from build123d import *

# Parameters (mm, degrees)
SKETCH_1_R          = 11
SKETCH_1_R_2        = 4.15
EXTRUDE_1_DEPTH     = 2
EXTRUDE_START       = 5
SKETCH_1_3_R        = 5.65
SKETCH_1_3_R_2      = 4.15
EXTRUDE_2_DEPTH     = 5
CUT_EXTRUDE_1_DEPTH = 4
SKETCH_4_R          = 11
SKETCH_4_R_2        = 6.15
EXTRUDE_3_DEPTH     = 10
CUT_EXTRUDE_START   = -8
SKETCH_5_W          = 5.562300803
SKETCH_5_H          = 5
CUT_EXTRUDE_2_DEPTH = 8


with BuildPart() as part:
    # Sketch 1 → Extrude 1 (new body)
    with BuildSketch(Plane(origin=(0, 0, 0), x_dir=(1, 0, 0), z_dir=(0, 1, 0))):
        with Locations(Location((0, 0, 0), (0, 0, 270))):
            Circle(SKETCH_1_R)
        with Locations(Location((0, 0, 0), (0, 0, 270))):
            Circle(SKETCH_1_R_2, mode=Mode.SUBTRACT)
    extrude(amount=-EXTRUDE_1_DEPTH)

    # Sketch 1_3 → Extrude 2 (add)
    with BuildSketch(Plane(origin=(0, 0, 0), x_dir=(1, 0, 0), z_dir=(0, 1, 0)).offset(EXTRUDE_START)):
        with Locations(Location((0, 0, 0), (0, 0, 270))):
            Circle(SKETCH_1_3_R)
        with Locations(Location((0, 0, 0), (0, 0, 270))):
            Circle(SKETCH_1_3_R_2, mode=Mode.SUBTRACT)
    extrude(amount=-EXTRUDE_2_DEPTH)

    # Sketch 2 → Cut-Extrude 1 (cut)
    with BuildSketch(Plane(origin=(0, 5, 0), x_dir=(1, 0, 0), z_dir=(0, 1, 0))):
        with BuildLine():
            Line((1.95, 5.302829433), (1.95, 3.663331817))
            ThreePointArc((1.95, 3.663331817), (4.15, 0), (1.95, -3.663331817))
            Line((1.95, -3.663331817), (1.95, -5.302829433))
            ThreePointArc((1.95, -5.302829433), (5.65, 0), (1.95, 5.302829433))
        make_face()
        with BuildLine():
            Line((-1.95, 5.302829433), (-1.95, 3.663331817))
            ThreePointArc((-1.95, 3.663331817), (-4.15, 0), (-1.95, -3.663331817))
            Line((-1.95, -3.663331817), (-1.95, -5.302829433))
            ThreePointArc((-1.95, -5.302829433), (-5.65, 0), (-1.95, 5.302829433))
        make_face()
    extrude(amount=-CUT_EXTRUDE_1_DEPTH, mode=Mode.SUBTRACT)

    # Sketch 4 → Extrude 3 (add)
    with BuildSketch(Plane.XZ.offset(2)):
        with Locations(Location((0, 0, 0), (0, 0, 90))):
            Circle(SKETCH_4_R)
        with Locations(Location((0, 0, 0), (0, 0, 270))):
            Circle(SKETCH_4_R_2, mode=Mode.SUBTRACT)
    extrude(amount=EXTRUDE_3_DEPTH)

    # Sketch 5 → Cut-Extrude 2 (cut)
    with BuildSketch(Plane.XZ.offset(12).offset(CUT_EXTRUDE_START)):
        with BuildLine():
            ThreePointArc((3.25, 10.508924778), (0, 11), (-3.25, 10.508924778))
            Line((-3.25, 10.508924778), (-3.25, 5.221110993))
            ThreePointArc((-3.25, 5.221110993), (0, 6.15), (3.25, 5.221110993))
            Line((3.25, 5.221110993), (3.25, 10.508924778))
        make_face()
        with Locations((-8.400091582, 0)):
            Rectangle(SKETCH_5_W, SKETCH_5_H)
    extrude(amount=CUT_EXTRUDE_2_DEPTH, mode=Mode.SUBTRACT)


solid = part.part
Geometry check sheet. Reference: the model listing, model coordinates, mm. A direction names the side the tool comes from. Round coordinates to 2 decimals unless told otherwise and drop trailing zeros. Order: outer loops, then holes, each group sorted by start corner. A loop starts at its lowest first (then second) coordinate and runs counter-clockwise, first axis right, second up. Notation, with made-up numbers: M 18.5,88.5 L 45.5,88.5 A14 cw 45.5,112.5 Z; hole C 14,-13 d5. An arc over 180 degrees is marked long. Answer in a Markdown table with one row per item. Add a question column.
Item 1: Draft check along Z on faces 1 (the face through (-1.95, 3, -4)), 2 (the face through (-8, -8, 2.5)). Enter one of: released by +Z, released by -Z, zero draft, split by the parting line, or undercut.
Item 2: Sectioned sample at B-B, the plane y = -5. Enter the section's corners in (x, z).
Item 3: Depth check by flat-ended pin: pin 1 Ø1.5 at (x, y) = (-8.5, -7) entering from +Z; pin 2 Ø6 at (y, z) = (-10, 8.5) entering from +X; pin 3 Ø0.5 at (y, z) = (2.5, 4.5) entering from -X; pin 4 Ø2 at (x, y) = (-0.5, -0.5) entering from +Z. Enter the tip coordinate at first touch or a pass-through.
Item 4: Sectioned sample at C-C, the plane z = -1.5. Enter the section's corners in (x, y).
Item 5: Sectioned sample at D-D, the plane y = 0.5. Enter the section's corners in (x, z), plus the area to 3 significant figures.
Item 6: Material ranges on L1, parallel to X at y = -3.75, z = 0; L2, parallel to Z at x = 0, y = 3, recorded low to high. Write a range as [from, to].
Item 7: Set-up check for faces 3 (the face through (-8, -4, 0)), 4 (the face through (1.847, -6.93, -5.866)), 5 (the face through (-3.25, -8, 8)): record each of +Z, -Z, +X, -X, +Y, -Y from which the full face is reachable in a straight line by a thin tool's end or side.
Item 8: Sectioned sample at A-A, the plane x = 0. Enter the section's corners in (y, z), plus the area to 3 significant figures.
Filled in:
| question | item | result |
|---|---|---|
| 1 | face 1 | zero draft |
| 1 | face 2 | undercut |
| 2 | outline | M -10.71,-2.5 A11 ccw long 3.25,10.51 L 3.25,5.22 A6.15 cw long -5.62,-2.5 Z; M -10.71,2.5 L -5.62,2.5 A6.15 cw -3.25,5.22 L -3.25,10.51 A11 ccw Z |
| 3 | pin 1 | stops at z = 7.81 |
| 3 | pin 2 | stops at x = 9.53 |
| 3 | pin 3 | stops at x = -1.95 |
| 3 | pin 4 | stops at z = 11 |
| 4 | outline | M -10.9,-4 L -5.96,-4 L -5.96,-2 L -3.87,-2 L -3.87,1 L -5.45,1 L -5.45,0 L -10.9,0 Z; M 3.87,-2 L 5.96,-2 L 5.96,-12 L 10.9,-12 L 10.9,0 L 5.45,0 L 5.45,1 L 3.87,1 Z |
| 5 | outline | C 0,0 d11.3; hole C 0,0 d8.3 |
| 5 | area | 46.2 mm² |
| 6 | L1 | x = [-11, -6.15], [6.15, 11] |
| 6 | L2 | z = [-5.65, -4.15], [4.15, 5.65] |
| 7 | face 3 | -X, -Y |
| 7 | face 4 | -Y |
| 7 | face 5 | +Z, -Y |
| 8 | outline | M -12,-11 L 0,-11 L 0,-5.65 L 5,-5.65 L 5,-4.15 L -2,-4.15 L -2,-6.15 L -12,-6.15 Z; M -4,6.15 L -2,6.15 L -2,4.15 L 5,4.15 L 5,5.65 L 0,5.65 L 0,11 L -4,11 Z |
| 8 | area | 101 mm² |
